Read the model definition and answer for the solid it produces. Units are mm, in the model's axes. A direction names the side the tool comes from. Coordinates: 2 decimals unless noted, no trailing zeros. Write each loop counter-clockwise with the first axis right and the second up, starting at its lowest first coordinate (ties: lowest second). Pieces come first, ordered by that corner, then holes. Notation, with made-up numbers: (2.25, -4.5) - (39.25, -4.5) arc R7 ccw to (39.25, 3.5) - close; hole circle Ø11 at (78, -33.5). An arc over 180 degrees is marked (long way). Return JSON: item names as keys, results as strings.
```python
from build123d import *
from build123d.topology import SkipClean

# Parameters (mm, degrees)
SKETCH4_W                       = 9.539179917
SKETCH4_H                       = 12.2
BOSS_EXTRUDE1_DEPTH             = 3
BOSS_EXTRUDE2_DEPTH             = 3
CIRPATTERN2_COUNT               = 4
CIRPATTERN2_COPY_1_DEPTH        = 3
CIRPATTERN2_COPY_2_DEPTH        = 3
CIRPATTERN2_COPY_3_DEPTH        = 3
CUT_EXTRUDE1_REACH              = 56.08
SKETCH8_R                       = 1.2
CUT_EXTRUDE1_DIRECTION_2_DEPTH  = 55.079941432
TAP_DRILL_FOR_M2X0_4_TAP1_D     = 1.6
TAP_DRILL_FOR_M2X0_4_TAP1_DEPTH = 3
M3_CLEARANCE_HOLE1_D            = 3.4
M3_CLEARANCE_HOLE1_DEPTH        = 3
M3_CLEARANCE_HOLE2_D            = 3.4
CIRPATTERN3_COUNT               = 4


with BuildPart() as part:
    # Sketch3 → Revolve1 (revolve)
    with BuildSketch(Plane.XY, mode=Mode.PRIVATE) as revolve1_sk:
        Polygon((2.25, 0), (2.25, 40.174859429), (7.25, 29.452324826), (7.25, 5), (18.652306326, 5), (20.983844617, 0), align=None)
    revolve(revolve1_sk.sketch.rotate(Axis((0, 21.429426471, 0), (0, -1, 0)), 180), axis=Axis((0, 21.429426471, 0), (0, -1, 0)))

    # Sketch4 → Boss-Extrude1 (add)
    with BuildSketch(Plane.XY.offset(0.5)):
        with Locations((8.440410041, -6.1)):
            Rectangle(SKETCH4_W, SKETCH4_H)
    boss_extrude1 = extrude(amount=BOSS_EXTRUDE1_DEPTH)

    # Mirror1: Boss-Extrude1 across plane
    add(boss_extrude1.mirror(Plane.XY))

    # Sketch9 → Boss-Extrude2 (add)
    with BuildSketch(Plane(origin=(-1.060660172, 0, 1.060660172), x_dir=(0, -1, 0), z_dir=(-0.7071067811865488, 0, 0.7071067811865464))):
        Polygon((0, 20.93016328), (18.126155741, 29.382528514), (24.465429667, 15.787911709), (0, 4.379494495), align=None)
    boss_extrude2 = extrude(amount=BOSS_EXTRUDE2_DEPTH)

    # Sketch10 → Cut-Revolve1 (revolve, cut)
    with SkipClean():  # the faces are left unmerged after this step: merging them gives an invalid solid
        with BuildSketch(Plane(origin=(0, 0, 0), x_dir=(-0.7071067811865464, 0, -0.7071067811865488), z_dir=(0.7071067811865488, 0, -0.7071067811865464)), mode=Mode.PRIVATE) as cut_revolve1_sk:
            Polygon((-2.25, 40.174859429), (-32.392261831, -24.465429667), (-32.392261831, 40.174859429), align=None)
        cut_revolve1 = revolve(cut_revolve1_sk.sketch.rotate(Axis((0, 55, 0), (0, -1, 0)), 315), axis=Axis((0, 55, 0), (0, -1, 0)), mode=Mode.SUBTRACT)

    # Mirror2: Boss-Extrude2, Cut-Revolve1 across plane
    with SkipClean():  # the faces are left unmerged after this step: merging them gives an invalid solid
        add(boss_extrude2.mirror(Plane(origin=(0, 0, 0), x_dir=(0.7071067811865465, 0, 0.7071067811865486), z_dir=(-0.7071067811865488, 0, 0.7071067811865464))))
        add(cut_revolve1.mirror(Plane(origin=(0, 0, 0), x_dir=(0.7071067811865465, 0, 0.7071067811865486), z_dir=(-0.7071067811865488, 0, 0.7071067811865464))), mode=Mode.SUBTRACT)

    # CirPattern2: Boss-Extrude2, Cut-Revolve1 ×4 about axis
    with SkipClean():  # the faces are left unmerged after this step: merging them gives an invalid solid
        cirpattern2_axis = Axis((0, 0, 0), (0, 1, 0))
        add([boss_extrude2.rotate(cirpattern2_axis, i * 360 / CIRPATTERN2_COUNT) for i in range(1, CIRPATTERN2_COUNT)])
        add([cut_revolve1.rotate(cirpattern2_axis, i * 360 / CIRPATTERN2_COUNT) for i in range(1, CIRPATTERN2_COUNT)], mode=Mode.SUBTRACT)

    # CirPattern2 copy 1 sketch → CirPattern2 copy 1 (add)
    with SkipClean():  # the faces are left unmerged after this step: merging them gives an invalid solid
        with BuildSketch(Plane(origin=(-1.060660172, 0, -1.060660172), x_dir=(0, -1, 0), z_dir=(-0.7071067811865465, 0, -0.707106781186549))):
            Polygon((0, -20.93016328), (18.126155741, -29.382528514), (24.465429667, -15.787911709), (0, -4.379494495), align=None)
        extrude(amount=CIRPATTERN2_COPY_1_DEPTH)

    # CirPattern2 copy 2 sketch → CirPattern2 copy 2 (add)
    with SkipClean():  # the faces are left unmerged after this step: merging them gives an invalid solid
        with BuildSketch(Plane(origin=(-1.060660172, 0, 1.060660172), x_dir=(0, -1, 0), z_dir=(-0.707106781186549, 0, 0.7071067811865465))):
            Polygon((0, -20.93016328), (18.126155741, -29.382528514), (24.465429667, -15.787911709), (0, -4.379494495), align=None)
        extrude(amount=CIRPATTERN2_COPY_2_DEPTH)

    # CirPattern2 copy 3 sketch → CirPattern2 copy 3 (add)
    with SkipClean():  # the faces are left unmerged after this step: merging them gives an invalid solid
        with BuildSketch(Plane(origin=(1.060660172, 0, 1.060660172), x_dir=(0, -1, 0), z_dir=(0.7071067811865465, 0, 0.7071067811865491))):
            Polygon((0, -20.93016328), (18.126155741, -29.382528514), (24.465429667, -15.787911709), (0, -4.379494495), align=None)
        extrude(amount=CIRPATTERN2_COPY_3_DEPTH)

    # CirPattern2 copy 4 sketch → CirPattern2 copy 4 (revolve, cut)
    with SkipClean():  # the faces are left unmerged after this step: merging them gives an invalid solid
        with BuildSketch(Plane(origin=(0, 0, 0), x_dir=(-0.7071067811865489, 0, 0.7071067811865464), z_dir=(0.7071067811865465, 0, 0.707106781186549))):
            Polygon((-2.25, -40.174859429), (-32.392261831, 24.465429667), (-32.392261831, -40.174859429), align=None)
        revolve(axis=Axis((0, 55, 0), (0, 1, 0)), mode=Mode.SUBTRACT)

    # CirPattern2 copy 5 sketch → CirPattern2 copy 5 (revolve, cut)
    with SkipClean():  # the faces are left unmerged after this step: merging them gives an invalid solid
        with BuildSketch(Plane(origin=(0, 0, 0), x_dir=(0.7071067811865464, 0, 0.7071067811865489), z_dir=(0.707106781186549, 0, -0.7071067811865465))):
            Polygon((-2.25, -40.174859429), (-32.392261831, 24.465429667), (-32.392261831, -40.174859429), align=None)
        revolve(axis=Axis((0, 55, 0), (0, 1, 0)), mode=Mode.SUBTRACT)

    # CirPattern2 copy 6 sketch → CirPattern2 copy 6 (revolve, cut)
    with SkipClean():  # the faces are left unmerged after this step: merging them gives an invalid solid
        with BuildSketch(Plane(origin=(0, 0, 0), x_dir=(0.7071067811865489, 0, -0.7071067811865462), z_dir=(-0.7071067811865465, 0, -0.7071067811865491))):
            Polygon((-2.25, -40.174859429), (-32.392261831, 24.465429667), (-32.392261831, -40.174859429), align=None)
        revolve(axis=Axis((0, 55, 0), (0, 1, 0)), mode=Mode.SUBTRACT)

    # Cut-Extrude1: up to this face of the body (flat: up to its plane)
    cut_extrude1_end = Plane(part.part.faces().sort_by_distance((8.458119385, -6.149603662, 0.5))[0])
    # Sketch8 → Cut-Extrude1 (cut, up to the picked face)
    with BuildSketch(Plane.XY.offset(3.5), mode=Mode.PRIVATE) as cut_extrude1_sk1:
        with Locations((10.21, -8.2)):
            Circle(SKETCH8_R)
    cut_extrude1_tool1 = split(extrude(cut_extrude1_sk1.sketch, amount=-CUT_EXTRUDE1_REACH, mode=Mode.PRIVATE), bisect_by=cut_extrude1_end, keep=Keep.BOTH, mode=Mode.PRIVATE)
    add(cut_extrude1_tool1.solids().sort_by(Axis((10.21, -8.2, 3.5), (0, 0, -1)))[0], mode=Mode.SUBTRACT)

    # Sketch8 → Cut-Extrude1 direction 2 (cut)
    with SkipClean():  # the faces are left unmerged after this step: merging them gives an invalid solid
        with BuildSketch(Plane.XY.offset(3.5)):
            with Locations((10.21, -8.2)):
                Circle(SKETCH8_R)
        extrude(amount=CUT_EXTRUDE1_DIRECTION_2_DEPTH, mode=Mode.SUBTRACT)

    # Tap Drill for M2x0.4 Tap1
    with Locations(Plane.XY.offset(-0.5)):
        with Locations((10.21, -8.2)):
            Hole(TAP_DRILL_FOR_M2X0_4_TAP1_D / 2, depth=TAP_DRILL_FOR_M2X0_4_TAP1_DEPTH)

    # M3 Clearance Hole1
    with Locations(Plane(origin=(-3.181980515, 0, 3.181980515), x_dir=(0.7071067811865465, 0, 0.7071067811865487), z_dir=(-0.7071067811865487, 0, 0.7071067811865465))):
        with Locations((14.998090227, -5.337914013), (19.976310592, -16.013742039)):
            m3_clearance_hole1 = Hole(M3_CLEARANCE_HOLE1_D / 2, depth=M3_CLEARANCE_HOLE1_DEPTH)

    # M3 Clearance Hole2 (through all)
    with Locations(Plane(origin=(1.060660172, 0, -1.060660172), x_dir=(0.7071067811865465, 0, 0.7071067811865487), z_dir=(-0.7071067811865487, 0, 0.7071067811865465))):
        with Locations((19.976310592, -16.013742039), (14.998090227, -5.337914013)):
            m3_clearance_hole2 = Hole(M3_CLEARANCE_HOLE2_D / 2)

    # CirPattern3: M3 Clearance Hole1, M3 Clearance Hole2 ×4 about axis
    with SkipClean():  # the faces are left unmerged after this step: merging them gives an invalid solid
        cirpattern3_axis = Axis((0, 55, 0), (0, -1, 0))
        add([m3_clearance_hole1.rotate(cirpattern3_axis, i * 360 / CIRPATTERN3_COUNT) for i in range(1, CIRPATTERN3_COUNT)], mode=Mode.SUBTRACT)
        add([m3_clearance_hole2.rotate(cirpattern3_axis, i * 360 / CIRPATTERN3_COUNT) for i in range(1, CIRPATTERN3_COUNT)], mode=Mode.SUBTRACT)


solid = part.part
```
(1) Determine the mould class of faces 1 (the face through (-8.591, -9.343, 14.955)), 2 (the face through (-12.972, -6.997, 8.759)), 3 (the face through (8, -12.2, -2)) for opening direction Y: +Y half, -Y half, draft (parallel to the pull), parting line (faces both ways), or undercut.
Answer:
{"face 1": "draft", "face 2": "undercut", "face 3": "-Y half"}
(2) A cutting plane is placed at A-A (y = -19.5). State how many separate pieces and enclosed holes the cut face has, and give its area (3 significant figures).
Answer:
{"separate pieces": "8", "enclosed holes": "0", "area": "311 mm²"}
(3) A cutting plane is placed at C-C (y = 36.5). Determine the outline of the cut face in (x, z).
Answer:
{"outline": "circle Ø7.93 at (0, 0); hole circle Ø4.5 at (0, 0)"}
(4) Which of the six approach directions +Z, -Z, +X, -X, +Y, -Y give full straight-line access (tool end or side, diameter ignored) to faces 4 (the face through (-8.835, -9.686, -15.199)), 5 (the face through (8, -12.2, 2)), 6 (the face through (-3.35, 17.05, 6.43)), 7 (the face through (11, -9.69, 13.12)), 8 (the face through (-15, 0, 0))?
Answer:
{"face 4": "-Z, -Y", "face 5": "+X, -X, -Y", "face 6": "+Y", "face 7": "-Y", "face 8": "-X, -Y"}
(5) A cutting plane is placed at B-B (y = 19). Determine the outline of the cut face in (x, z).
Answer:
{"outline": "circle Ø14.5 at (0, 0); hole circle Ø4.5 at (0, 0)"}
(6) Straight lines are drawn through the part: line 1 (X direction, y = -8.2, z = -2.85); line 2 (X direction, y = -8.2, z = 14); line 3 (Z direction, x = -13.5, y = -0.5). For each, find the intervals that lie inside material, in ascending order. Write a range as from..to.
Answer:
{"line 1": "-9.21..-8.75, 3.67..9.41, 11.01..13.21", "line 2": "-20.36..-16.12, -11.88..-7.64, 7.64..9.01, 11.41..11.88, 16.12..20.36", "line 3": "-16.37..-15.62, -11.38..-7.14, 7.14..11.38, 15.62..16.37"}
(7) Flat-ended cylindrical pins translate along their axes: P1, Ø6, axis at x = 3.5, y = 0.5, coming from the +Z side; P2, Ø9.5, axis at x = 7.5, z = 5, coming from the -Y side; P3, Ø6, axis at x = 0, z = 0, coming from the -Y side; P4, Ø10, axis at x = 16.5, y = -18, coming from the +Z side. Find the tip coordinate at first contact, or state that the pin passes through.
Answer:
{"P1": "z = 20.98", "P2": "y = -19.75", "P3": "y = 0", "P4": "z = 23.79"}
